Here's how the part is built. I have some questions about the finished solid (model axes, mm). A direction names the side the tool comes from. Give positions to 0.01 mm unless a question says otherwise; leave off trailing zeros. Loops run counter-clockwise (first coordinate to the right, second up) from the corner with the lowest first, then second, coordinate; pieces in that order, holes last.
Q1. For faces 4 (the face through (-1.08, -4.88, 1.97)), 5 (the face through (0.867, -3.905, -0.521)), 6 (the face through (1, -2.2, 4)), which set-ups out of +Z, -Z, +X, -X, +Y, -Y let a thin tool reach every point of the face, with its end or its side?
Q2. We'd pull the mould along Y, two halves only. Please class faces 1 (the face through (1.19, -5.37, -0.99)), 2 (the face through (-2, -2, 1)), 3 (the face through (-1.6, -4.9, 0)): +Y half, -Y half, draft (parallel to the pull), parting line (faces both ways), or undercut.
Q3. If we section it at A-A (y = 0): Please give me the cut outline in (x, z), plus the area to 3 significant figures.
Q4. I need wall thicknesses on line 1 (Y direction, x = 0, z = -0.6); line 2 (Y direction, x = 0, z = 3.3); line 3 (Y direction, x = -3, z = 3.75). Which ranges of each line are inside material? Lowest first, please.
Q5. Will these pins go through, and if not, where does the flat tip stop? P1, Ø4, axis at x = 1, y = 1, coming from the -Z side; P2, Ø1.5, axis at y = 1.5, z = 2.5, coming from the +X side.
Q6. If we section it at D-D (x = -3.75): Please give me the cut outline in (y, z).
Q7. If we section it at C-C (z = 1.25): Please give me the cut outline in (x, y).
from build123d import *

# Parameters (mm, degrees)
SKETCH_1_R          = 5
EXTRUDE_1_DEPTH     = 4
SKETCH_2_R          = 5.5
EXTRUDE_2_DEPTH     = 2
SKETCH_3_R          = 2.1
CUT_EXTRUDE_1_DEPTH = 10.823441352
SKETCH_4_R          = 4
CUT_EXTRUDE_2_DEPTH = 3


with BuildPart() as part:
    # ｽｹｯﾁ1 → ﾎﾞｽ - 押し出し1 (new body)
    with BuildSketch(Plane.XY):
        Circle(SKETCH_1_R)
    extrude(amount=EXTRUDE_1_DEPTH)

    # ｽｹｯﾁ2 → ﾎﾞｽ - 押し出し2 (add)
    with BuildSketch(Plane(origin=(0, 0, 0), x_dir=(-1, 0, 0), z_dir=(0, 0, -1))):
        Circle(SKETCH_2_R)
    extrude(amount=EXTRUDE_2_DEPTH)

    # ｽｹｯﾁ3 → ｶｯﾄ - 押し出し1 (cut, through all)
    with BuildSketch(Plane.XY.offset(4)):
        Circle(SKETCH_3_R)
    extrude(amount=-CUT_EXTRUDE_1_DEPTH, mode=Mode.SUBTRACT)

    # ｽｹｯﾁ4 → ｶｯﾄ - 押し出し2 (cut)
    with BuildSketch(Plane(origin=(0, 0, -2), x_dir=(-1, 0, 0), z_dir=(0, 0, -1))):
        Circle(SKETCH_4_R)
    extrude(amount=-CUT_EXTRUDE_2_DEPTH, mode=Mode.SUBTRACT)


solid = part.part
Check sheet entries:
1. face 4: +Z
1. face 5: -Z
1. face 6: +Z, +X, -X, +Y, -Y
2. face 1: parting line
2. face 2: undercut
2. face 3: draft
3. outline: (-5.5, -2) - (-4, -2) - (-4, 1) - (-2.1, 1) - (-2.1, 4) - (-5, 4) - (-5, 0) - (-5.5, 0) - close; (2.1, 1) - (4, 1) - (4, -2) - (5.5, -2) - (5.5, 0) - (5, 0) - (5, 4) - (2.1, 4) - close
3. area: 25.4 mm2
4. line 1: y = -5.5 to -4, 4 to 5.5
4. line 2: y = -5 to -2.1, 2.1 to 5
4. line 3: y = -4 to 4
5. P1: stops at z = 1
5. P2: stops at x = 4.94
6. outline: (-4.02, -2) - (-1.39, -2) - (-1.39, 1) - (1.39, 1) - (1.39, -2) - (4.02, -2) - (4.02, 0) - (3.31, 0) - (3.31, 4) - (-3.31, 4) - (-3.31, 0) - (-4.02, 0) - close
7. outline: circle Ø10 at (0, 0); hole circle Ø4.2 at (0, 0)
